Input: part model. Units: mm. Frame: model coordinates. Face numbers are marked on the shaded views. A direction names the side the tool comes from. Give positions to 0.01 mm unless a question says otherwise; leave off trailing zeros. Write each loop counter-clockwise with the first axis right and the second up, starting at its lowest first coordinate (ties: lowest second). Pieces come first, ordered by that corner, then holes.
```python
from build123d import *

# Parameters (mm, degrees)
F0_R     = 9.75
F1_DEPTH = 15
F2_R     = 3.25
F3_DEPTH = 125
F4_R     = 1.5
F5_DEPTH = 8


with BuildPart() as f1:
    # F0 (on Top) → F1 (new body)
    with BuildSketch(Plane.XY):
        Polygon((34, 14), (-14, 14), (-14, -14), (134, -14), (134, 14), (134, 32), (129, 32), (129, 14), (89, 14), (89, 32), (79, 32), (79, 14), (39, 14), (39, 32), (34, 32), align=None)
        Circle(F0_R, mode=Mode.SUBTRACT)
        with Locations((40, 0)):
            Circle(F0_R, mode=Mode.SUBTRACT)
        with Locations((80, 0)):
            Circle(F0_R, mode=Mode.SUBTRACT)
        with Locations((120, 0)):
            Circle(F0_R, mode=Mode.SUBTRACT)
    extrude(amount=F1_DEPTH)

    # F2 (on face) → F3 (cut)
    with BuildSketch(Plane.YZ.offset(134)):
        with Locations((26.161687, 7.5)):
            Circle(F2_R)
    extrude(amount=-F3_DEPTH, mode=Mode.SUBTRACT)

    # F4 (on face) → F5 (cut)
    with BuildSketch(Plane.XZ.offset(14)):
        with Locations((120, 7.5)):
            Circle(F4_R)
        with Locations((80, 7.5)):
            Circle(F4_R)
        with Locations((40, 7.5)):
            Circle(F4_R)
        with Locations((0, 7.5)):
            Circle(F4_R)
    extrude(amount=-F5_DEPTH, mode=Mode.SUBTRACT)


solid = f1.part
```
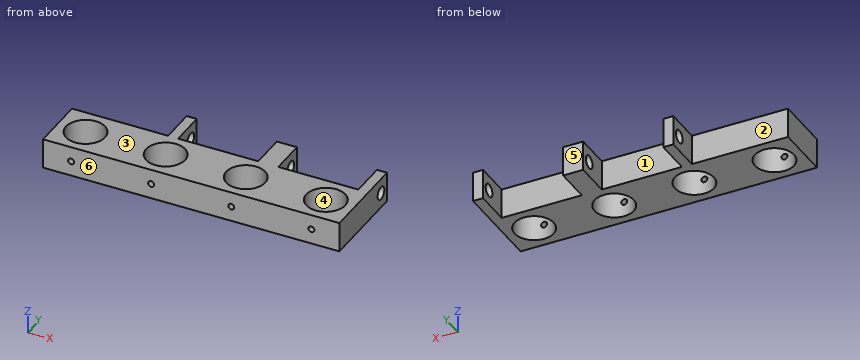
Item 1: Ray query, line 1 (X direction, y = 25.5, z = 13); line 2 (X direction, y = -11.4, z = 7.5); line 3 (Y direction, x = 85.5, z = 6). Return the intervals inside material, ascending.
Item 2: Set-up query: the marked faces 1, 2 and 3. Return all of +Z, -Z, +X, -X, +Y, -Y with unobstructed straight access to the full face (end or side cutting, diameter ignored); none if empty.
Item 3: Section D-D (x = 116.5). Return loops of the section in (y, z), and give its area (3 significant figures).
Item 4: Pin query (flat end, axial travel): pin 1 (7.5 mm diameter, centred on y = 23.5, z = 7.5, fed in from -X); pin 2 (7.5 mm diameter, centred on x = 5, z = 11, fed in from +Y); pin 3 (5 mm diameter, centred on x = 76.5, y = 12.5, fed in from -Z); pin 4 (15.5 mm diameter, centred on x = 120, y = 0, fed in from -Z). Return the tip coordinate at first contact, or that it passes through.
Item 5: Section B-B (x = 0). Return loops of the section in (y, z), and give its area (3 significant figures).
Item 6: Section A-A (y = 0). Return loops of the section in (x, z), and give its area (3 significant figures).
Item 7: Section C-C (z = 2.5). Return loops of the section in (x, y).
Item 8: Mould query, pull axis Y, two halves, no side actions, for the marked faces 4, 5 and 6. Classes: +Y half, -Y half, draft (parallel to the pull), parting line (faces both ways), or undercut.
Solved:
1. line 1: x = 34 to 39, 79 to 89, 129 to 134
1. line 2: x = -14 to -1.5, 1.5 to 38.5, 41.5 to 78.5, 81.5 to 118.5, 121.5 to 134
1. line 3: y = -14 to -8.05, 8.05 to 23.28, 29.04 to 32
2. face 1: +Z, -Z, +Y
2. face 2: +Z, -Z, -X, +Y
2. face 3: +Z, +X, -X, +Y, -Y
3. outline: (-14, 0) - (-9.1, 0) - (-9.1, 15) - (-14, 15) - close; (9.1, 0) - (14, 0) - (14, 15) - (9.1, 15) - close
3. area: 147 mm2
4. pin 1: stops at x = 34
4. pin 2: stops at y = 14
4. pin 3: stops at z = 0
4. pin 4: passes through
5. outline: (-14, 0) - (-9.75, 0) - (-9.75, 6) - (-14, 6) - close; (-14, 9) - (-9.75, 9) - (-9.75, 15) - (-14, 15) - close; (9.75, 0) - (14, 0) - (14, 15) - (9.75, 15) - close
5. area: 115 mm2
6. outline: (-14, 0) - (-9.75, 0) - (-9.75, 15) - (-14, 15) - close; (9.75, 0) - (30.25, 0) - (30.25, 15) - (9.75, 15) - close; (49.75, 0) - (70.25, 0) - (70.25, 15) - (49.75, 15) - close; (89.75, 0) - (110.25, 0) - (110.25, 15) - (89.75, 15) - close; (129.75, 0) - (134, 0) - (134, 15) - (129.75, 15) - close
6. area: 1,050 mm2
7. outline: (-14, -14) - (134, -14) - (134, 32) - (129, 32) - (129, 14) - (89, 14) - (89, 32) - (79, 32) - (79, 14) - (39, 14) - (39, 32) - (34, 32) - (34, 14) - (-14, 14) - close; hole circle Ø19.5 at (0, 0); hole circle Ø19.5 at (40, 0); hole circle Ø19.5 at (80, 0); hole circle Ø19.5 at (120, 0)
8. face 4: undercut
8. face 5: +Y half
8. face 6: -Y half
